Geometry check sheet. Reference: drawing and pictorial views, mm from the part's lowest x, y, z. A direction names the side the tool comes from. Give positions to 0.01 mm unless a question says otherwise; leave off trailing zeros. Write each loop counter-clockwise with the first axis right and the second up, starting at its lowest first coordinate (ties: lowest second). Pieces come first, ordered by that corner, then holes.
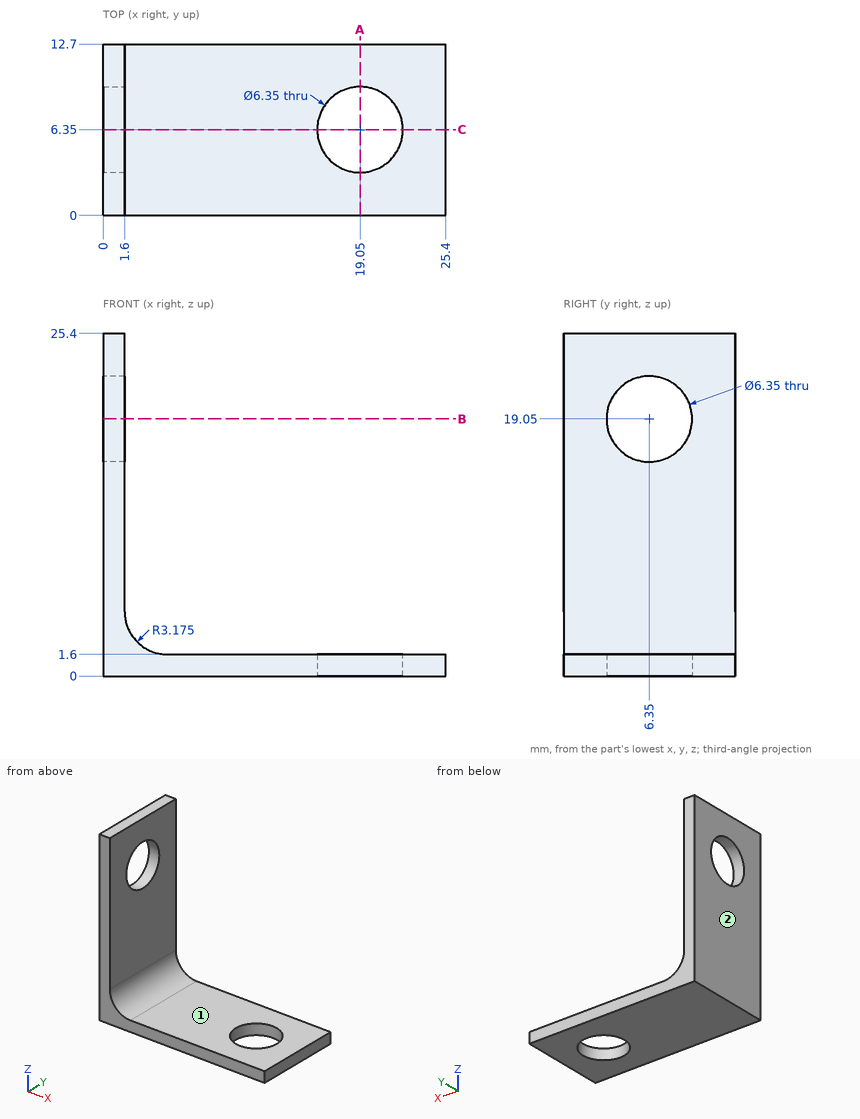
Item 1: Sectioned sample at C-C on y = 6.35. State how many separate pieces and enclosed holes the cut face has.
Answer key:
separate pieces: 3
enclosed holes: 0
Item 2: Depth check by flat-ended pin: pin 1 (10 mm diameter, centred on x = 7, z = 10, fed in from -Y); pin 2 (4 mm diameter, centred on y = 2.5, z = 6.5, fed in from +X); pin 3 (4 mm diameter, centred on x = 12, y = 4.5, fed in from +Z). Enter the tip coordinate at first touch or a pass-through.
Answer key:
pin 1: passes through
pin 2: stops at x = 1.61
pin 3: stops at z = 1.6
Item 3: Set-up check for the marked faces 1 and 2: record each of +Z, -Z, +X, -X, +Y, -Y from which the full face is reachable in a straight line by a thin tool's end or side.
Answer key:
face 1: +Z, +X, +Y, -Y
face 2: +Z, -Z, -X, +Y, -Y
Item 4: Sectioned sample at A-A on x = 19.05. Record the cut outline in (y, z) (1 decimal).
Answer key:
outline: (0, 0) - (3.2, 0) - (3.2, 1.6) - (0, 1.6) - close; (9.5, 0) - (12.7, 0) - (12.7, 1.6) - (9.5, 1.6) - close
Item 5: Scan lines: line 1 along Z through (x, y) = (0.9, 6.35) (3 decimals); line 2 along Y through (x, z) = (19.05, 0.95) (3 decimals); line 3 along Z through (x, y) = (21.75, 10.5). Record each from-to range of solid material in increasing order.
Answer key:
line 1: z = 0 to 15.875, 22.225 to 25.4
line 2: y = 0 to 3.175, 9.525 to 12.7
line 3: z = 0 to 1.6
Item 6: Sectioned sample at B-B on z = 19.05. Record the cut outline in (x, y) (1 decimal), then the cut area to 3 significant figures.
Answer key:
outline: (0, 0) - (1.6, 0) - (1.6, 3.2) - (0, 3.2) - close; (0, 9.5) - (1.6, 9.5) - (1.6, 12.7) - (0, 12.7) - close
area: 10.2 mm2
